from build123d import *

# Parameters (mm, degrees)
SKETCH1_W                  = 76.2
SKETCH1_H                  = 25.4
BOSS_EXTRUDE1_DEPTH        = 19.05
SKETCH2_W                  = 69.85
SKETCH2_H                  = 12.7
CUT_EXTRUDE1_DEPTH         = 83.55
M6X1_0_TAPPED_HOLE1_D      = 5
F_9_0_196_DIAMETER_HOLE1_D = 4.9784


with BuildPart() as part:
    # Sketch1 → Boss-Extrude1 (new body)
    with BuildSketch(Plane(origin=(0, 0, 0), x_dir=(1, 0, 0), z_dir=(0, 1, 0))):
        with Locations((-38.1, 12.7)):
            Rectangle(SKETCH1_W, SKETCH1_H)
    extrude(amount=BOSS_EXTRUDE1_DEPTH)

    # Sketch2 → Cut-Extrude1 (cut, through all)
    with BuildSketch(Plane.XY):
        with Locations((-34.925, 12.7)):
            Rectangle(SKETCH2_W, SKETCH2_H)
    extrude(amount=-CUT_EXTRUDE1_DEPTH, mode=Mode.SUBTRACT)

    # M6x1.0 Tapped Hole1 (through all)
    with Locations(Plane.ZY.offset(76.2)):
        with Locations((-12.7, 12.7)):
            Hole(M6X1_0_TAPPED_HOLE1_D / 2)

    # #9 (0.196) Diameter Hole1 (through all)
    with Locations(Plane(origin=(0, 6.35, 0), x_dir=(1, 0, 0), z_dir=(0, 1, 0))):
        with Locations((-45.72, 12.7), (-7.62, 12.7)):
            Hole(F_9_0_196_DIAMETER_HOLE1_D / 2)


solid = part.part
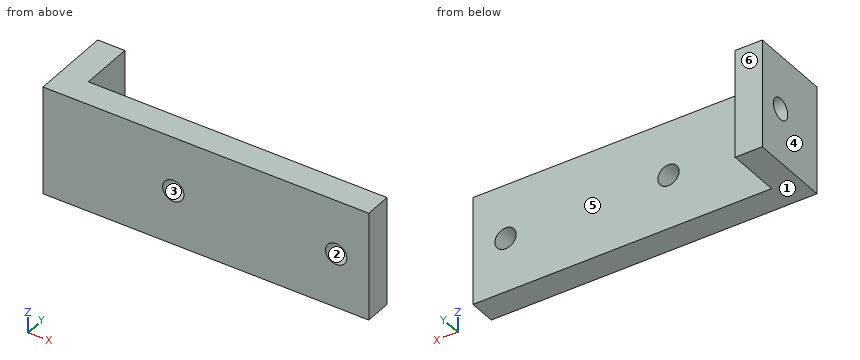
Source: CAD feature listing. Evaluate the final solid. Frame: model axes, mm. Face numbers are marked on the shaded views. A direction names the side the tool comes from. Round coordinates to 2 decimals unless told otherwise and drop trailing zeros. Order: outer loops, then holes, each group sorted by start corner. A loop starts at its lowest first (then second) coordinate and runs counter-clockwise, first axis right, second up. Notation, with made-up numbers: (-4, 1.25) -> (34, 1.25) arc R24 cw to (34, 23.25) -> close; hole circle Ø11 at (-6.75, -5). An arc over 180 degrees is marked (long way). Answer as CSV lines item,"result".
Item 1: Line query: L1, parallel to X at y = 2.5, z = -12.7; L2, parallel to Y at x = -73.5, z = -12.7; L3, parallel to Z at x = -45.72, y = 3.5. Output: solid intervals per line, ascending.
A:
L1,"-76.2 to -48.21, -43.23 to -10.11, -5.13 to 0"
L2,"0 to 10.2, 15.2 to 19.05"
L3,"-25.4 to -15.19, -10.21 to 0"
Item 2: Pin query (flat end, axial travel): pin 1 Ø6 at (x, z) = (-19.5, -3.5) entering from +Y; pin 2 Ø5 at (y, z) = (3.5, -3) entering from +X; pin 3 Ø4 at (y, z) = (10, -12.5) entering from +X. Return the tip coordinate at first contact, or that it passes through.
A:
pin 1,"y = 6.35"
pin 2,"x = 0"
pin 3,"x = -69.85"
Item 3: Section B-B, the plane y = 12.7. Return loops of the section in (x, z), plus the area to 3 significant figures.
A:
outline,"(-76.2, -25.4) -> (-69.85, -25.4) -> (-69.85, -15.2) -> (-76.2, -15.2) -> close; (-76.2, -10.2) -> (-69.85, -10.2) -> (-69.85, 0) -> (-76.2, 0) -> close"
area,"130 mm²"
Item 4: Section A-A, the plane x = -7.62. Return loops of the section in (y, z).
A:
outline,"(0, -25.4) -> (6.35, -25.4) -> (6.35, -15.19) -> (0, -15.19) -> close; (0, -10.21) -> (6.35, -10.21) -> (6.35, 0) -> (0, 0) -> close"
Item 5: Reachability of the marked faces 5 and 6 from +Z, -Z, +X, -X, +Y, -Y: full face, straight path, thin tool, end or side. Return the list, or none.
A:
face 5,"+Z, -Z, +X, +Y"
face 6,"+Z, -Z, +X, -X, +Y"
Item 6: Section D-D, the plane z = -23.5. Return loops of the section in (x, y), plus the area to 3 significant figures.
A:
outline,"(-76.2, 0) -> (0, 0) -> (0, 6.35) -> (-69.85, 6.35) -> (-69.85, 19.05) -> (-76.2, 19.05) -> close"
area,"565 mm²"
Item 7: Pull-direction query (Z, two-part tool) for the marked faces 1, 2, 3 and 4; classes: pulls with the +Z half, pulls with the -Z half, needs draft (parallel to the pull), parting line crosses it, or undercut.
A:
face 1,"pulls with the -Z half"
face 2,"undercut"
face 3,"undercut"
face 4,"needs draft"
Item 8: Section C-C, the plane y = 2. Return loops of the section in (x, z).
A:
outline,"(-76.2, -25.4) -> (0, -25.4) -> (0, 0) -> (-76.2, 0) -> close; hole circle Ø4.98 at (-45.72, -12.7); hole circle Ø4.98 at (-7.62, -12.7)"
